Can you work these out from the model? Positions are in its coordinate system, mm. A direction names the side the tool comes from. Give positions to 0.01 mm unless a question says otherwise; leave off trailing zeros. Order: outer loops, then holes, each group sorted by start corner. A loop starts at its lowest first (then second) coordinate and runs counter-clockwise, first axis right, second up. Notation, with made-up numbers: M 74,19 L 106,19 A25 cw 106,52 Z; hole C 62.25,-22.5 d9. An arc over 180 degrees is marked long. Answer as a JSON object with one key per item and string values.
```python
from build123d import *

# Parameters (mm, degrees)
MAIN_BODY_DEPTH             = 22.55
RUBBER_BEARING_SLEEVE_DEPTH = 18.5
BOSS_EXTRUDE3_DEPTH         = 19.05
M5X0_8_TAPPED_HOLE1_D       = 4.2
M5X0_8_TAPPED_HOLE1_DEPTH   = 16
M5X0_8_TAPPED_HOLE1_TIP     = 1.2618073


with BuildPart() as part:
    # Sketch1 → Main Body (new, symmetric)
    with BuildSketch(Plane(origin=(0, 0, 0), x_dir=(1, 0, 0), z_dir=(0, 1, 0))):
        with BuildLine():
            Line((-20.975, 12), (-20.975, -9.4))
            Line((-20.975, -9.4), (-22.5, -10.925))
            Line((-22.5, -10.925), (-22.5, -19.9))
            Line((-22.5, -19.9), (-10.675, -19.9))
            Line((-10.675, -19.9), (-9.675, -18.9))
            Line((-9.675, -18.9), (9.675, -18.9))
            Line((9.675, -18.9), (10.675, -19.9))
            Line((10.675, -19.9), (22.5, -19.9))
            Line((22.5, -19.9), (22.5, -10.925))
            Line((22.5, -10.925), (20.975, -9.4))
            Line((20.975, -9.4), (20.975, 12))
            Line((20.975, 12), (8.333560049, 12))
            Line((8.333560049, 12), (7.981030265, 11.502310894))
            ThreePointArc((7.981030265, 11.502310894), (0, -14), (-7.981030265, 11.502310894))
            Line((-7.981030265, 11.502310894), (-8.333560049, 12))
            Line((-8.333560049, 12), (-20.975, 12))
        make_face()
    extrude(amount=MAIN_BODY_DEPTH, both=True)

    # Sketch1<3> → Rubber Bearing Sleeve (add, symmetric)
    with BuildSketch(Plane(origin=(0, 0, 0), x_dir=(1, 0, 0), z_dir=(0, 1, 0))):
        with BuildLine():
            Line((-4.624138726, 6.528195849), (-8.092242771, 11.424342735))
            ThreePointArc((-8.092242771, 11.424342735), (-6.430730954, -12.435662403), (14, 0))
            ThreePointArc((14, 0), (12.435662403, 6.430730954), (8.092242771, 11.424342735))
            Line((8.092242771, 11.424342735), (4.624138726, 6.528195849))
            ThreePointArc((4.624138726, 6.528195849), (7.106092802, 3.674703402), (8, 0))
            ThreePointArc((8, 0), (-3.674703402, -7.106092802), (-4.624138726, 6.528195849))
        make_face()
    extrude(amount=RUBBER_BEARING_SLEEVE_DEPTH, both=True)

    # Sketch1<4> → Boss-Extrude3 (add, symmetric)
    with BuildSketch(Plane(origin=(0, 0, 0), x_dir=(1, 0, 0), z_dir=(0, 1, 0))):
        Polygon((-20.275, 12.5), (-20.275, 12), (-8.333560049, 12), (-5.188313398, 7.559651787), (-4.780301158, 7.848660458), (-8.075, 12.5), align=None)
        Polygon((8.333560049, 12), (20.275, 12), (20.275, 12.5), (8.075, 12.5), (4.780301158, 7.848660458), (5.188313398, 7.559651787), align=None)
    extrude(amount=BOSS_EXTRUDE3_DEPTH, both=True)

    # M5x0.8 Tapped Hole1
    with Locations(Plane.XY.offset(19.9)):
        with Locations((-16.05, 15.05), (16.05, 15.05), (16.05, -15.05), (-16.05, -15.05)):
            Hole(M5X0_8_TAPPED_HOLE1_D / 2, depth=M5X0_8_TAPPED_HOLE1_DEPTH)
            with Locations((0, 0, -(M5X0_8_TAPPED_HOLE1_DEPTH + M5X0_8_TAPPED_HOLE1_TIP / 2))):  # 118° drill point
                Cone(0, M5X0_8_TAPPED_HOLE1_D / 2, M5X0_8_TAPPED_HOLE1_TIP, mode=Mode.SUBTRACT)


solid = part.part
```
1) Thinking about a two-plate mould opening in X: for faces 4 (the face through (20.8, 0.1, -12)), 5 (the face through (0, 18.5, 10)), 6 (the face through (-22.5, 0, 15)), which applies, pulls with the +X half, pulls with the -X half, needs draft (parallel to the pull), parting line crosses it, or undercut?
Results found:
{"face 4": "needs draft", "face 5": "undercut", "face 6": "pulls with the -X half"}
2) I'm going to push flat-ended pins straight in: pin 1 Ø0.6 at (y, z) = (4, -12.5) entering from +X (3 decimals); pin 2 Ø6 at (x, z) = (5.5, 10.5) entering from -Y; pin 3 Ø1.5 at (x, y) = (9, 0) entering from +Z (3 decimals); pin 4 Ø1 at (x, y) = (5, 13.5) entering from +Z. Where does each tip first touch, or does it pass through?
Results found:
{"pin 1": "stops at x = 20.275", "pin 2": "stops at y = -22.55", "pin 3": "stops at z = 18.975", "pin 4": "stops at z = 18.9"}
3) For faces 1 (the face through (0, 0, 18.9)), 2 (the face through (11.9, 19.05, -12.2)), 3 (the face through (-20.975, 0, -1)), which set-ups out of +Z, -Z, +X, -X, +Y, -Y let a thin tool reach every point of the face, with its end or its side?
Results found:
{"face 1": "+Z, +Y, -Y", "face 2": "-Z, +Y", "face 3": "-Z, -X, +Y, -Y"}
4) I want a section at C-C on x = 0. Write out the boundary of the cut face in (y, z).
Results found:
{"outline": "M -22.55,14 L -18.5,14 L -18.5,8 L 18.5,8 L 18.5,14 L 22.55,14 L 22.55,18.9 L -22.55,18.9 Z"}
5) I want a section at B-B on y = -7. Write out the boundary of the cut face in (x, z) (3 decimals).
Results found:
{"outline": "M -22.5,10.925 L -20.975,9.4 L -20.975,-12 L -20.275,-12 L -20.275,-12.5 L -8.075,-12.5 L -4.78,-7.849 L -5.188,-7.56 L -7.981,-11.502 A14 cw -8.092,-11.424 L -4.624,-6.528 A8 cw long 4.624,-6.528 L 8.092,-11.424 A14 cw 7.981,-11.502 L 5.188,-7.56 L 4.78,-7.849 L 8.075,-12.5 L 20.275,-12.5 L 20.275,-12 L 20.975,-12 L 20.975,9.4 L 22.5,10.925 L 22.5,19.9 L 10.675,19.9 L 9.675,18.9 L -9.675,18.9 L -10.675,19.9 L -22.5,19.9 Z"}
6) I want a section at A-A on z = 0. Write out the boundary of the cut face in (x, y) (3 decimals).
Results found:
{"outline": "M -20.975,-22.55 L -14,-22.55 L -14,-18.5 L -8,-18.5 L -8,18.5 L -14,18.5 L -14,22.55 L -20.975,22.55 Z; M 8,-18.5 L 14,-18.5 L 14,-22.55 L 20.975,-22.55 L 20.975,22.55 L 14,22.55 L 14,18.5 L 8,18.5 Z"}
7) I want a section at D-D on z = 13. Write out the boundary of the cut face in (x, y), and give its area (3 significant figures).
Results found:
{"outline": "M -22.5,-22.55 L -5.2,-22.55 L -5.2,-18.5 L 5.2,-18.5 L 5.2,-22.55 L 22.5,-22.55 L 22.5,22.55 L 5.2,22.55 L 5.2,18.5 L -5.2,18.5 L -5.2,22.55 L -22.5,22.55 Z; hole C -16.05,-15.05 d4.2; hole C -16.05,15.05 d4.2; hole C 16.05,-15.05 d4.2; hole C 16.05,15.05 d4.2", "area": "1,890 mm²"}
8) I need wall thicknesses on L1, parallel to Y at x = -16.05, z = 16.25; L2, parallel to X at y = -15, z = 16; L3, parallel to Z at x = 5, y = 10 (3 decimals). Which ranges of each line are inside material? Lowest first, please.
Results found:
{"L1": "y = -22.55 to -17.15, -12.95 to 12.95, 17.15 to 22.55", "L2": "x = -22.5 to -18.15, -13.95 to 13.95, 18.15 to 22.5", "L3": "z = -8.159 to -7.693, -7.059 to -6.245, 6.245 to 18.9"}
